Design review of the part shown in the three views and the two pictorial views. Dimensions are in mm from the part's minimum x, y and z. Coordinates: 2 decimals unless noted, no trailing zeros. Loops run counter-clockwise (first coordinate to the right, second up) from the corner with the lowest first, then second, coordinate; pieces in that order, holes last. Notation, with made-up numbers: M -3,41 L 46,41 A32 cw 46,69 Z; hole C 24.25,-11 d9. An arc over 180 degrees is marked long. Answer as a JSON object with one key per item and string values. Group by question number.
Item 1: Add section B-B (y = 180.5). State the section outline as (x, z) points, then the cut area to 3 significant figures.
Item 2: Wall thickness on L1, parallel to Y at x = 41, z = 6; L2, parallel to Y at x = 57.5, z = 0.75; L3, parallel to Y at x = 177.5, z = 5.5: over which ranges is each line inside the solid? List them lowest first. Write a range as from..to.
Item 3: Insertion check: pin 1 (4 mm diameter, centred on y = 179, z = 5, fed in from -X). The pin has a flat end and moves straight along its axis. Give the tip position at first contact, or say it passes through.
Item 4: Add section C-C (z = 1.5). Count the separate pieces of the cut face and the enclosed holes in it, then the cut area to 3 significant figures.
Item 5: Add section A-A (x = 133.5). State the section outline as (y, z) points.
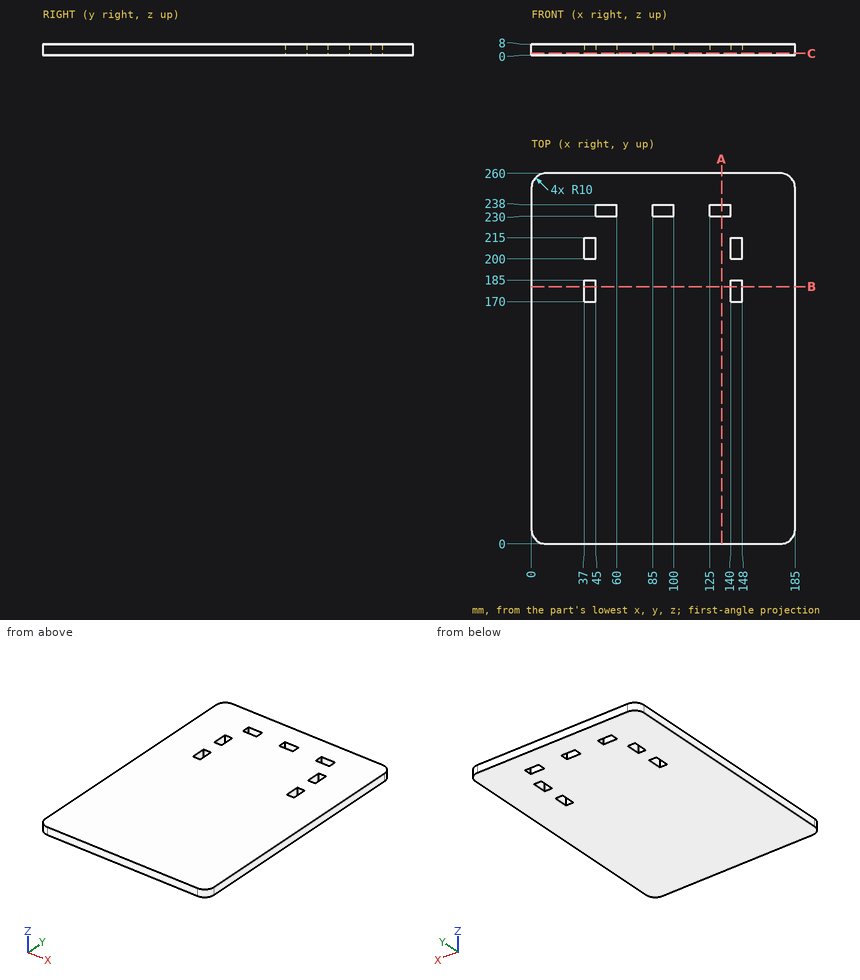
From the geometry:
{
 "1": {"outline": "M 0,0 L 37,0 L 37,8 L 0,8 Z; M 45,0 L 140,0 L 140,8 L 45,8 Z; M 148,0 L 185,0 L 185,8 L 148,8 Z", "area": "1,350 mm²"},
 "2": {"L1": "y = 0..170, 185..200, 215..260", "L2": "y = 0..230, 238..260", "L3": "y = 0.32..259.68"},
 "3": {"pin 1": "stops at x = 0"},
 "4": {"separate pieces": "1", "enclosed holes": "7", "area": "47,200 mm²"},
 "5": {"outline": "M 0,0 L 230,0 L 230,8 L 0,8 Z; M 238,0 L 260,0 L 260,8 L 238,8 Z"}
}
